The figure shows three views and two pictorial views of one solid part (mm, origin at its lowest corner). Answer the questions. Coordinates: 2 decimals unless noted, no trailing zeros. Order: outer loops, then holes, each group sorted by start corner. A loop starts at its lowest first (then second) coordinate and runs counter-clockwise, first axis right, second up. Notation, with made-up numbers: (-27.5, 33) - (14.5, 33) arc R20 ccw to (14.5, 59) - close; hole circle Ø3 at (-19.75, -6). An arc over 180 degrees is marked (long way). Use one line per item in the form item = value. Start each with the question number.
Item 1: Section B-B, the plane x = 55 is taken. Write down the section's boundary in (y, z), and give its area (3 significant figures).
Item 2: Each of these flat-tipped pins is pushed along its axis until it touches: pin 1 Ø3 at (x, y) = (4, 11) entering from -Z; pin 2 Ø1.5 at (x, z) = (124.5, 1.5) entering from -Y. Where does it stop, or does it pass through?
Item 3: Consider line 1 along Y through (x, z) = (55, 1.2); line 2 along X through (y, z) = (3.75, 2.1); line 3 along Y through (x, z) = (4, 1.7). Determine where each line is inside the solid, lowest interval first. Write a range as [from, to].
Item 4: Section A-A, the plane y = 4 is taken. Write down the section's boundary in (x, z), and give its area (3 significant figures).
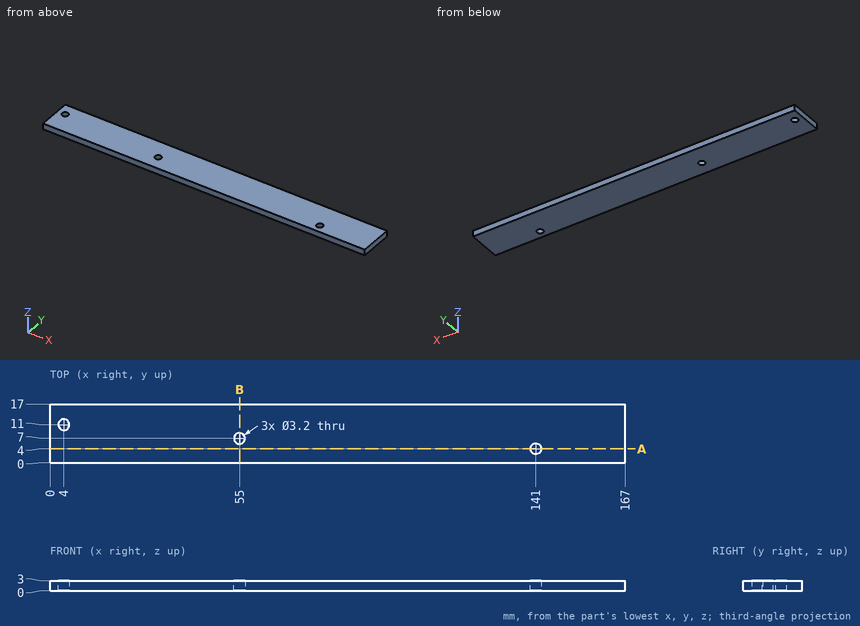
Response:
q1.outline = (0, 0) - (5.4, 0) - (5.4, 3) - (0, 3) - close; (8.6, 0) - (17, 0) - (17, 3) - (8.6, 3) - close
q1.area = 41.4 mm2
q2.pin_1 = through
q2.pin_2 = 0
q3.line_1 = [0, 5.4], [8.6, 17]
q3.line_2 = [0, 139.42], [142.58, 167]
q3.line_3 = [0, 9.4], [12.6, 17]
q4.outline = (0, 0) - (139.4, 0) - (139.4, 3) - (0, 3) - close; (142.6, 0) - (167, 0) - (167, 3) - (142.6, 3) - close
q4.area = 491 mm2
